Source: CAD feature listing. Evaluate the final solid. Frame: model axes, mm. A direction names the side the tool comes from. Coordinates: 2 decimals unless noted, no trailing zeros. Loops run counter-clockwise (first coordinate to the right, second up) from the corner with the lowest first, then second, coordinate; pieces in that order, holes last.
from build123d import *

# Parameters (mm, degrees)
F1_DEPTH = 44.45
F2_DEPTH = 12.7


with BuildPart() as f1:
    # F0 (on Front) → F1 (new body)
    with BuildSketch(Plane.XZ):
        with BuildLine():
            ThreePointArc((-113.546669, -12.471259), (-119.864514, -6.759491), (-114.816669, 0.100445))
            Line((-114.816669, 0.100445), (-114.816669, 2.230411))
            Line((-114.816669, 2.230411), (-113.546669, 2.230411))
            Line((-113.546669, 2.230411), (-113.546669, 16.103741))
            Line((-113.546669, 16.103741), (-123.071669, 16.103741))
            Line((-123.071669, 16.103741), (-123.071669, -28.346259))
            Line((-123.071669, -28.346259), (-113.546669, -28.346259))
            Line((-113.546669, -28.346259), (-113.546669, -12.471259))
        make_face()
        with BuildLine():
            ThreePointArc((-112.276669, 0.100445), (-107.228825, -6.759491), (-113.546669, -12.471259))
            Line((-113.546669, -12.471259), (-113.546669, -28.346259))
            Line((-113.546669, -28.346259), (-104.021669, -28.346259))
            Line((-104.021669, -28.346259), (-104.021669, 16.103741))
            Line((-104.021669, 16.103741), (-113.546669, 16.103741))
            Line((-113.546669, 16.103741), (-113.546669, 2.230411))
            Line((-113.546669, 2.230411), (-112.276669, 2.230411))
            Line((-112.276669, 2.230411), (-112.276669, 0.100445))
        make_face()
        with BuildLine():
            Line((-113.546669, -6.121259), (-113.546669, -12.471259))
            ThreePointArc((-113.546669, -12.471259), (-107.228825, -6.759491), (-112.276669, 0.100445))
            Line((-112.276669, 0.100445), (-112.276669, 2.230411))
            Line((-112.276669, 2.230411), (-113.546669, 2.230411))
            Line((-113.546669, 2.230411), (-113.546669, -6.121259))
        make_face()
        with BuildLine():
            Line((-114.816669, 2.230411), (-114.816669, 0.100445))
            ThreePointArc((-114.816669, 0.100445), (-119.864514, -6.759491), (-113.546669, -12.471259))
            Line((-113.546669, -12.471259), (-113.546669, -6.121259))
            Line((-113.546669, -6.121259), (-113.546669, 2.230411))
            Line((-113.546669, 2.230411), (-114.816669, 2.230411))
        make_face()
    extrude(amount=F1_DEPTH)

    # F0 (on Front) → F2 (cut)
    with BuildSketch(Plane.XZ):
        with BuildLine():
            Line((-113.546669, -6.121259), (-113.546669, -12.471259))
            ThreePointArc((-113.546669, -12.471259), (-107.228825, -6.759491), (-112.276669, 0.100445))
            Line((-112.276669, 0.100445), (-112.276669, 2.230411))
            Line((-112.276669, 2.230411), (-113.546669, 2.230411))
            Line((-113.546669, 2.230411), (-113.546669, -6.121259))
        make_face()
        with BuildLine():
            Line((-114.816669, 2.230411), (-114.816669, 0.100445))
            ThreePointArc((-114.816669, 0.100445), (-119.864514, -6.759491), (-113.546669, -12.471259))
            Line((-113.546669, -12.471259), (-113.546669, -6.121259))
            Line((-113.546669, -6.121259), (-113.546669, 2.230411))
            Line((-113.546669, 2.230411), (-114.816669, 2.230411))
        make_face()
    extrude(amount=F2_DEPTH, mode=Mode.SUBTRACT)


solid = f1.part
Q1. Access query for faces 1 (the flat face through (-113, -22, 16.104)), 2 (the flat face through (-114, -12.7, -7)). Directions: +Z, -Z, +X, -X, +Y, -Y. A direction counts if a zero-diameter tool reaches every point of the face in a straight line with its end or side. Return the directions, or none.
Q2. Section B-B, the plane x = -108.25. Return the cut outline in (y, z).
Q3. Line query: line 1 along Y through (x, z) = (-114, -11); line 2 along Z through (x, y) = (-110.5, -9); line 3 along Z through (x, y) = (-111.75, -3). Output: solid intervals per line, ascending.
Q4. Section A-A, the plane y = -4. Return the cut outline in (x, z), plus the area to 3 significant figures.
Q5. Contact query for a flat-ended pin moving along its axis: pin 1 Ø10 at (x, z) = (-114.5, -4) entering from +Y. Output: stop coordinate, or through.
Q6. Draft query along Z for faces 3 (the flat face through (-114, -6, 2.23)), 4 (the flat face through (-114, -22, -28.346)), 5 (the flat face through (-104.022, -22, -6)). Return one class per face: +Z half, -Z half, draft (parallel to the pull), parting line (faces both ways), or undercut.
Q7. Section C-C, the plane x = -116.25. Return the cut outline in (y, z), plus the area to 3 significant figures.
Derived:
1. face 1: +Z, +X, -X, +Y, -Y
1. face 2: +Y
2. outline: (-44.45, -28.35) - (0, -28.35) - (0, -9.62) - (-12.7, -9.62) - (-12.7, -2.62) - (0, -2.62) - (0, 16.1) - (-44.45, 16.1) - close
3. line 1: y = -44.45 to -12.7
3. line 2: z = -28.35 to -11.69, -0.55 to 16.1
3. line 3: z = -28.35 to -12.21, -0.03 to 16.1
4. outline: (-123.07, -28.35) - (-104.02, -28.35) - (-104.02, 16.1) - (-123.07, 16.1) - close; hole (-114.82, 0.1) arc R6.35 ccw (long way) to (-112.28, 0.1) - (-112.28, 2.23) - (-114.82, 2.23) - close
4. area: 715 mm2
5. pin 1: stops at y = 0
6. face 3: undercut
6. face 4: -Z half
6. face 5: draft
7. outline: (-44.45, -28.35) - (0, -28.35) - (0, -11.87) - (-12.7, -11.87) - (-12.7, -0.38) - (0, -0.38) - (0, 16.1) - (-44.45, 16.1) - close
7. area: 1,830 mm2
